Autodesk Inventor part; units mm, degrees
ref_plane "YZ Plane" through (0, 0, 0) normal (1, 0, 0) x (0, 1, 0)
ref_plane "XZ Plane" through (0, 0, 0) normal (0, 1, 0) x (-1, 0, 0)
ref_plane "XY Plane" through (0, 0, 0) normal (0, 0, 1) x (1, 0, 0)
sketch "Boceto1" plane through (0, 0, 0) normal (0, 1, 0) x (-1, 0, 0)
  line L0 (-19.9533, 14.4643) -> (7.0467, 14.4643)
  line L1 (7.0467, 14.4643) -> (7.0467, -12.5357)
  line L2 (7.0467, -12.5357) -> (-19.9533, -12.5357)
  line L3 (-19.9533, -12.5357) -> (-19.9533, 14.4643)
  point P0 (0, 0)
  dimension "d0" = 27
  dimension "d1" = 27
extrude "Extrusión1" add sketch "Boceto1" along normal blind 62
sketch "Boceto2" plane through (0, 62, 0) normal (0, 1, 0) x (1, 0, 0)
  line L0 (-7.0467, -14.4643) -> (19.9533, -14.4643)
  line L1 (19.9533, -14.4643) -> (19.9533, 12.5357)
  line L2 (19.9533, 12.5357) -> (-7.0467, 12.5357)
  line L3 (-7.0467, 12.5357) -> (-7.0467, -14.4643)
  line L4 (-1.0467, 6.5357) -> (13.9533, 6.5357)
  line L5 (13.9533, 6.5357) -> (13.9533, -8.4643)
  line L6 (13.9533, -8.4643) -> (-1.0467, -8.4643)
  line L7 (-1.0467, -8.4643) -> (-1.0467, 6.5357)
  point P0 (0, 0)
  dimension "d4" = 6
  dimension "d5" = 6
  dimension "d6" = 6
  dimension "d7" = 6
extrude "Extrusión2" cut sketch "Boceto2" against normal blind 31 contours L4 L5 L6 L7
sketch "Boceto3" plane through (19.9533, 0, -12.5357) normal (0, 0, -1) x (-1, 0, 0)
  line L0 (27, 0) -> (0, 0)
  line L1 (27, 0) -> (27, 62)
  line L2 (0, 0) -> (0, 62)
  line L3 (20, 25) -> (7, 25)
  line L4 (7, 25) -> (7, 0)
  line L5 (7, 0) -> (20, 0)
  line L6 (20, 0) -> (20, 25)
  line L7 (0, 62) -> (27, 62)
  circle A0 centre (13.5, 39) radius 2.55
  point P0 (19.9533, 0)
  dimension "d10" = 7
  dimension "d11" = 7
  dimension "d12" = 25
  dimension "d16" = 5.1
  dimension "d17" = 13.5
  dimension "d18" = 23
extrude "Extrusión3" cut sketch "Boceto3" against normal blind 30 contours L0 L4 L3 L6
sketch "Boceto4" plane through (19.9533, 62, -12.5357) normal (0, 0, -1) x (-1, 0, 0)
  line L0 (0, -62) -> (0, 0)
  circle A0 centre (13.5, -25) radius 1.55
  line L1 (21, -31) -> (6, -31)
  point P0 (19.9533, -62)
  dimension "d19" = 3.1
  dimension "d20" = 13.5
  dimension "d34" = 6
extrude "Extrusión4" cut sketch "Boceto4" against normal blind 7
sketch "Boceto5" plane through (-7.0467, 62, 14.4643) normal (0, 0, 1) x (1, 0, 0)
  line L0 (27, -62) -> (27, 0)
  circle A0 centre (13.5, -25) radius 7.75
  line L1 (21, -31) -> (6, -31)
  point P0 (7.0467, -62)
  dimension "d24" = 15.5
  dimension "d25" = 13.5
  dimension "d33" = 6
extrude "Extrusión5" cut sketch "Boceto5" against normal blind 3
sketch "Boceto6" plane through (6.4533, 37, 11.4643) normal (0, 0, 1) x (1, 0, 0)
  circle A0 centre (0, 0) radius 7.75
  circle A1 centre (0, 0) radius 5.65
  point P0 (-6.4533, -37)
  dimension "d29" = 11.3
extrude "Extrusión6" cut sketch "Boceto6" against normal blind 3 contours A1
sketch "Boceto8" plane through (-7.0467, 0, -12.5357) normal (-1, 0, 0) x (0, 0, 1)
  line L0 (27, 0) -> (27, 62)
  circle A0 centre (13.5, 37) radius 1.5
  line L1 (0, 25) -> (27, 25)
  line L2 (0, 25) -> (27, 25)
  point P0 (12.5357, 0)
  dimension "d42" = 13.5
  dimension "d43" = 3
  dimension "d47" = 12
extrude "Extrusión8" cut sketch "Boceto8" against normal through all
sketch "Boceto10" plane through (0, 31, 0) normal (0, 1, 0) x (1, 0, 0)
  line L0 (-1.0467, 6.5357) -> (13.9533, 6.5357)
  line L1 (13.9533, 6.5357) -> (13.9533, -8.4643)
  circle A0 centre (6.4533, -0.9643) radius 1.5
  point P0 (0, 0)
  dimension "d62" = 3
  dimension "d63" = 7.5
  dimension "d64" = 7.5
extrude "Extrusión10" cut sketch "Boceto10" against normal through all
properties part number "Cubeta Final sin huecos"
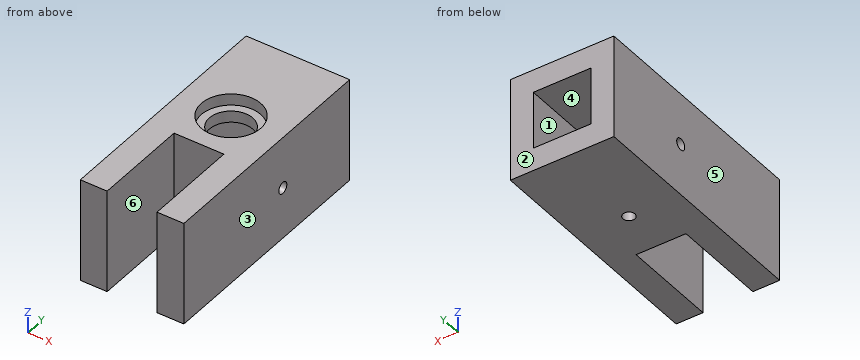
The model under review builds one solid part; all positions refer to its coordinate system, in mm. Face numbers are marked on the shaded views. A direction names the side the tool comes from. Round coordinates to 2 decimals unless told otherwise and drop trailing zeros. Loops run counter-clockwise (first coordinate to the right, second up) from the corner with the lowest first, then second, coordinate; pieces in that order, holes last. Notation, with made-up numbers: (44.5, 22) - (48.5, 22) arc R27 cw to (48.5, 57) - close; hole circle Ø11 at (-10, -9.75). An arc over 180 degrees is marked (long way). Write each question's results on one line, items separated by ' | '. Start each with the question number.
Q1. Take a section at D-D on z = 3.5. Give the boundary of the cut face in (x, y), plus the area to 3 significant figures.
Q2. Take a section at B-B on y = 19.5. Give the boundary of the cut face in (x, z).
Q3. Take a section at C-C on x = 6.75. Give the boundary of the cut face in (y, z), plus the area to 3 significant figures.
Q4. Insertion check: P1, Ø4.5, axis at x = 6, y = 33.5, coming from the +Z side; P2, Ø1.9, axis at x = 6.45, y = 37, coming from the +Z side; P3, Ø3, axis at x = 2, z = -8, coming from the -Y side; P4, Ø4, axis at x = 6.45, z = 0.96, coming from the +Y side. Each pin has a flat end and moves straight along its axis. Give the tip position at first contact, or say it passes through.
Q5. Draft analysis for pull direction X (two halves, no side actions). For the marked faces 1, 2 and 3, state which applies: pulls with the +X half, pulls with the -X half, needs draft (parallel to the pull), parting line crosses it, or undercut.
Q6. Tool access review of the marked faces 4, 5 and 6: name each direction out of +Z, -Z, +X, -X, +Y, -Y from which nothing blocks a thin tool from reaching the whole face with its end or side.
Q7. Take a section at A-A on y = 37. Give the boundary of the cut face in (x, z).
Q8. Wall thickness on line 1 along Z through (x, y) = (10.75, 57.5); line 2 along X through (y, z) = (37, 12.9); line 3 along X through (y, z) = (35, 5.25): over which ranges is each line inside the solid? List them lowest first. Write a range as [from, to].
Data:
1) outline: (-7.05, 0) - (-0.05, 0) - (-0.05, 25) - (12.95, 25) - (12.95, 0) - (19.95, 0) - (19.95, 62) - (13.95, 62) - (13.95, 31) - (-1.05, 31) - (-1.05, 62) - (-7.05, 62) - close | area: 884 mm²
2) outline: (-7.05, -12.54) - (-0.05, -12.54) - (-0.05, 14.46) - (-7.05, 14.46) - close; (12.95, -12.54) - (19.95, -12.54) - (19.95, 14.46) - (12.95, 14.46) - close
3) outline: (25, -12.54) - (35.48, -12.54) - (35.48, -6.54) - (31, -6.54) - (31, -0.51) - (25, -0.51) - close; (25, 2.43) - (31, 2.43) - (31, 8.46) - (31.36, 8.46) - (31.36, 11.46) - (29.26, 11.46) - (29.26, 14.46) - (25, 14.46) - close; (38.52, -12.54) - (62, -12.54) - (62, -6.54) - (38.52, -6.54) - close; (42.64, 8.46) - (62, 8.46) - (62, 14.46) - (44.74, 14.46) - (44.74, 11.46) - (42.64, 11.46) - close | area: 418 mm²
4) P1: stops at z = 11.46 | P2: passes through | P3: stops at y = 25 | P4: stops at y = 31
5) face 1: undercut | face 2: needs draft | face 3: pulls with the +X half
6) face 4: +Y | face 5: +Z, -Z, -X, +Y, -Y | face 6: +Z, -Z, -Y
7) outline: (-7.05, -12.54) - (4.9, -12.54) - (4.9, -6.54) - (-1.05, -6.54) - (-1.05, -0.54) - (-7.05, -0.54) - close; (-7.05, 2.46) - (-1.05, 2.46) - (-1.05, 8.46) - (0.8, 8.46) - (0.8, 11.46) - (-1.3, 11.46) - (-1.3, 14.46) - (-7.05, 14.46) - close; (8, -12.54) - (19.95, -12.54) - (19.95, -0.54) - (13.95, -0.54) - (13.95, -6.54) - (8, -6.54) - close; (12.1, 8.46) - (13.95, 8.46) - (13.95, 2.46) - (19.95, 2.46) - (19.95, 14.46) - (14.2, 14.46) - (14.2, 11.46) - (12.1, 11.46) - close
8) line 1: z = [-12.54, -6.54], [8.46, 14.46] | line 2: x = [-7.05, -1.3], [14.2, 19.95] | line 3: x = [-7.05, -1.05], [13.95, 19.95]
